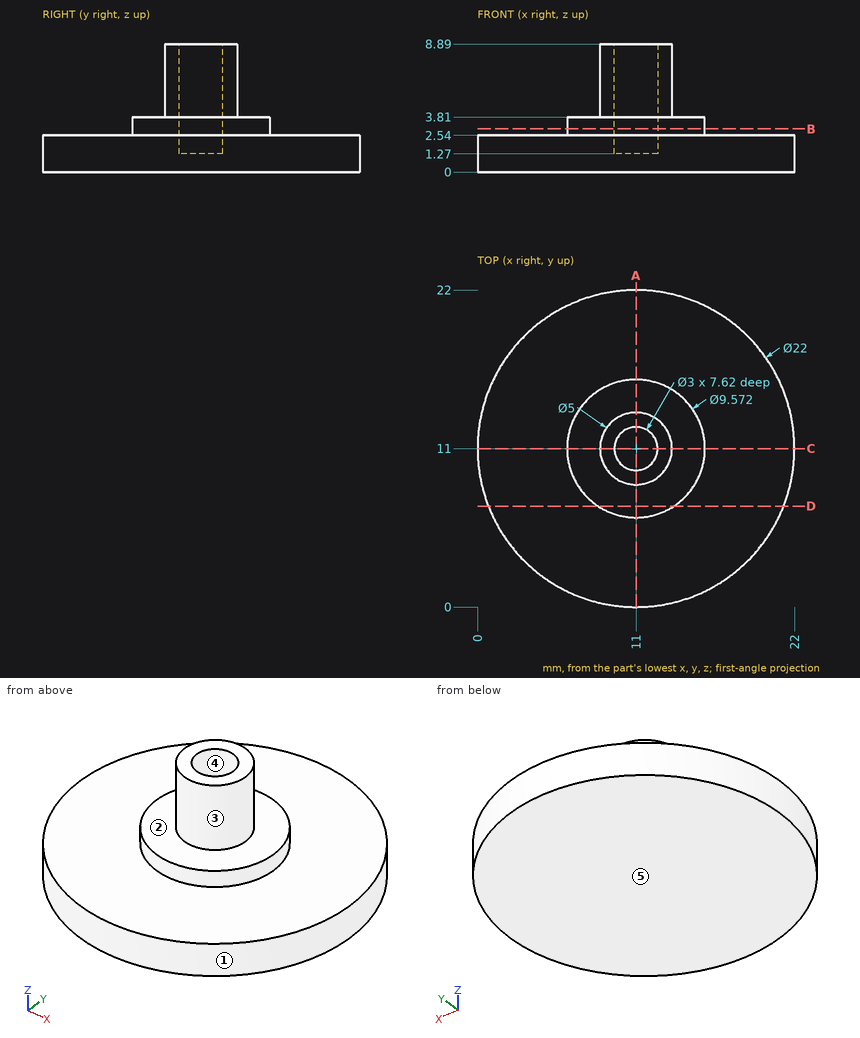
Part print with two shaded views. Sizes in mm from the minimum x, y, z corner. A direction names the side the tool comes from. Give positions to 0.01 mm unless a question says otherwise; leave off trailing zeros. Order: outer loops, then holes, each group sorted by start corner. A loop starts at its lowest first (then second) coordinate and runs counter-clockwise, first axis right, second up.
1) Mould opens along X. For the marked faces 3, 4 and 5 say: +X half, -X half, draft (parallel to the pull), parting line (faces both ways), or undercut.
2) Saw through at A-A, the plane x = 11. Write the cut outline in (y, z), then the cut area to 3 significant figures.
3) Saw through at D-D, the plane y = 7. Write the cut outline in (x, z), then the cut area to 3 significant figures.
4) Pin check, flat tips, straight feed: pin 1 (10 mm diameter, centred on x = 4.5, y = 19.5, fed in from +Z); pin 2 (0.9 mm diameter, centred on x = 10.5, y = 11, fed in from +Z); pin 3 (5 mm diameter, centred on x = 15, z = 4, fed in from -Y). Stop position of each tip, or through.
5) 3-axis set-ups, long thin cutter, end or side, ignore diameter. For the marked faces 1 and 2: which of +Z, -Z, +X, -X, +Y, -Y reach the whole face in a straight line?
6) Saw through at B-B, the plane z = 3. Write the cut outline in (x, y).
7) Wall check: probe 1 along Y at (x, z) = (11, 5); probe 2 along Y at (x, z) = (11, 3.25); probe 3 along X at (y, z) = (12, 3). Give the ranges that are in metal, low to high.
Computed:
1. face 3: parting line
1. face 4: undercut
1. face 5: draft
2. outline: (0, 0) - (22, 0) - (22, 2.54) - (15.79, 2.54) - (15.79, 3.81) - (13.5, 3.81) - (13.5, 8.89) - (12.5, 8.89) - (12.5, 1.27) - (9.5, 1.27) - (9.5, 8.89) - (8.5, 8.89) - (8.5, 3.81) - (6.21, 3.81) - (6.21, 2.54) - (0, 2.54) - close
2. area: 70.6 mm2
3. outline: (0.75, 0) - (21.25, 0) - (21.25, 2.54) - (13.63, 2.54) - (13.63, 3.81) - (8.37, 3.81) - (8.37, 2.54) - (0.75, 2.54) - close
3. area: 58.7 mm2
4. pin 1: stops at z = 2.54
4. pin 2: stops at z = 1.27
4. pin 3: stops at y = 0.18
5. face 1: +Z, -Z
5. face 2: +Z
6. outline: circle Ø9.57 at (11, 11); hole circle Ø3 at (11, 11)
7. probe 1: y = 8.5 to 9.5, 12.5 to 13.5
7. probe 2: y = 6.21 to 9.5, 12.5 to 15.79
7. probe 3: x = 6.32 to 9.88, 12.12 to 15.68
